```python
from build123d import *

# Parameters (mm, degrees)
BOSS_EXTRUDE1_DEPTH     = 15
SKETCH7_R               = 12.1
CUT_EXTRUDE3_DEPTH      = 71.5
SKETCH8_R               = 12.1
CUT_EXTRUDE4_DEPTH      = 71.5
CUT_EXTRUDE4_DEPTH_BACK = 71.5
BOSS_EXTRUDE4_DEPTH     = 8
BOSS_EXTRUDE5_DEPTH     = 2
SKETCH11_R              = 2.75
CUT_EXTRUDE5_DEPTH      = 24
SKETCH12_R              = 6
CUT_EXTRUDE6_DEPTH      = 4
CHAMFER1_SIZE           = 4
CUT_EXTRUDE7_DEPTH      = 28


with BuildPart() as part:
    # Sketch1 → Boss-Extrude1 (new body)
    with BuildSketch(Plane.XY):
        with BuildLine():
            Line((-23, -30.39874498), (-32, -30.39874498))
            Line((-32, -30.39874498), (-32, -39.99874498))
            Line((-32, -39.99874498), (-23, -39.99874498))
            ThreePointArc((-23, -39.99874498), (0, -46.14), (23, -39.99874498))
            Line((23, -39.99874498), (32, -39.99874498))
            Line((32, -39.99874498), (32, -30.39874498))
            Line((32, -30.39874498), (23, -30.39874498))
            Line((23, -30.39874498), (23, 39.99874498))
            ThreePointArc((23, 39.99874498), (0, 46.14), (-23, 39.99874498))
            Line((-23, 39.99874498), (-23, -30.39874498))
        make_face()
    extrude(amount=BOSS_EXTRUDE1_DEPTH)

    # Sketch7 → Cut-Extrude3 (cut)
    with BuildSketch(Plane.ZY.offset(23)):
        with Locations((0, 22.49874498)):
            Circle(SKETCH7_R)
    extrude(amount=-CUT_EXTRUDE3_DEPTH, mode=Mode.SUBTRACT)

    # Sketch8 → Cut-Extrude4 (cut, two sides)
    with BuildSketch(Plane.ZY.offset(23)) as cut_extrude4_sk:
        with Locations((0, -22.49874498)):
            Circle(SKETCH8_R)
    extrude(amount=CUT_EXTRUDE4_DEPTH, mode=Mode.SUBTRACT)
    extrude(cut_extrude4_sk.sketch, amount=-CUT_EXTRUDE4_DEPTH_BACK, mode=Mode.SUBTRACT)

    # Sketch9 → Boss-Extrude4 (add)
    with BuildSketch(Plane.ZY.offset(23)):
        with BuildLine():
            Line((0, 34.59874498), (0, 32.99874498))
            ThreePointArc((0, 32.99874498), (10.5, 22.49874498), (0, 11.99874498))
            Line((0, 11.99874498), (0, 10.39874498))
            ThreePointArc((0, 10.39874498), (12.1, 22.49874498), (0, 34.59874498))
        make_face()
    boss_extrude4 = extrude(amount=-BOSS_EXTRUDE4_DEPTH)

    # Sketch10 → Boss-Extrude5 (add)
    with BuildSketch(Plane.ZY.offset(32)):
        with BuildLine():
            Line((0, -32.99874498), (0, -34.59874498))
            ThreePointArc((0, -34.59874498), (5.040833264, -33.49874498), (9.16515139, -30.39874498))
            Line((9.16515139, -30.39874498), (6.916646586, -30.39874498))
            ThreePointArc((6.916646586, -30.39874498), (3.69459064, -32.327274881), (0, -32.99874498))
        make_face()
    boss_extrude5 = extrude(amount=-BOSS_EXTRUDE5_DEPTH)

    # Mirror1: Boss-Extrude4, Boss-Extrude5 across plane
    add(boss_extrude4.mirror(Plane(origin=(0, 0, 0), x_dir=(0, 0, 1), z_dir=(1, 0, 0))))
    add(boss_extrude5.mirror(Plane(origin=(0, 0, 0), x_dir=(0, 0, 1), z_dir=(1, 0, 0))))

    # Sketch11 → Cut-Extrude5 (cut)
    with BuildSketch(Plane(origin=(0, 0, 0), x_dir=(-1, 0, 0), z_dir=(0, 0, -1))):
        Circle(SKETCH11_R)
        with Locations((0, 41.14108798)):
            Circle(SKETCH11_R)
        with Locations((0, -41.14108798)):
            Circle(SKETCH11_R)
    extrude(amount=-CUT_EXTRUDE5_DEPTH, mode=Mode.SUBTRACT)

    # Sketch12 → Cut-Extrude6 (cut)
    with BuildSketch(Plane.XY.offset(15)):
        Circle(SKETCH12_R)
        with Locations((0, -41.14108798)):
            Circle(SKETCH12_R)
        with Locations((0, 41.14108798)):
            Circle(SKETCH12_R)
    extrude(amount=-CUT_EXTRUDE6_DEPTH, mode=Mode.SUBTRACT)

    # Chamfer1
    chamfer1_edges = [part.edges().sort_by_distance(p)[0] for p in [
        (-13.591823685, 44.092651643, 15),
        (13.591823685, 44.092651643, 15),
        (13.591823685, -44.092651643, 15),
        (27.5, -39.99874498, 15),
        (32, -39.99874498, 7.5),
        (-13.591823685, -44.092651643, 15),
        (-27.5, -39.99874498, 15),
        (-32, -39.99874498, 7.5),
    ]]
    chamfer(chamfer1_edges, length=CHAMFER1_SIZE)

    # Sketch13 → Cut-Extrude7 (cut)
    with BuildSketch(Plane.XY.offset(15)):
        Polygon((31.8, -38.311994276), (31.8, -30.59874498), (22.8, -30.59874498), (22.8, 43.889056734), (37.227618098, 33.583615236), (38.561263468, -37.220829882), align=None)
        Polygon((-37.227618098, 33.583615236), (-38.561263468, -37.220829882), (-31.8, -38.311994276), (-31.8, -30.59874498), (-22.8, -30.59874498), (-22.8, 43.889056734), align=None)
    extrude(amount=-CUT_EXTRUDE7_DEPTH, mode=Mode.SUBTRACT)


solid = part.part
```
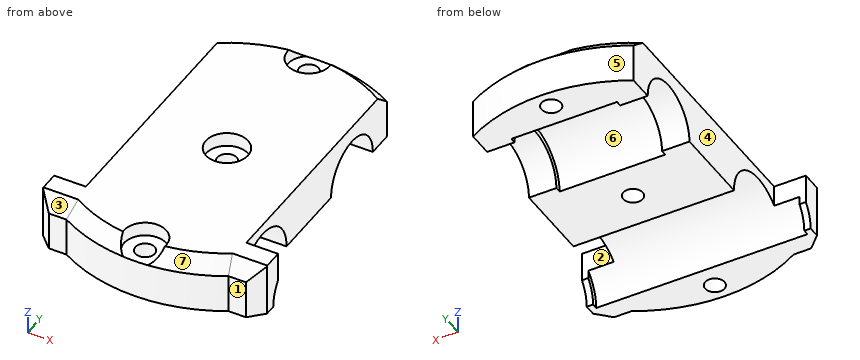
CAD build for the part. Positions are in the model's coordinates, mm. Face numbers are marked on the shaded views. A direction names the side the tool comes from. Round coordinates to 2 decimals unless told otherwise and drop trailing zeros. Loops run counter-clockwise (first coordinate to the right, second up) from the corner with the lowest first, then second, coordinate; pieces in that order, holes last. Notation, with made-up numbers: M 35,-35.5 L 59,-35.5 A21 ccw 59,-14.5 Z; hole C 4,19 d6. An arc over 180 degrees is marked long. Return JSON: item names as keys, results as strings. Group by question number.
(1) Drop flat-ended pins along their axis: P1, Ø7.5, axis at y = -2, z = 5.5, coming from the -X side; P2, Ø6.5, axis at x = 27, z = 12, coming from the +Y side; P3, Ø9, axis at x = -2.5, y = -40, coming from the +Z side; P4, Ø8, axis at y = -3, z = 12.5, coming from the +X side. Give the stop position or say it passes through.
(2) Saw through at C-C, the plane x = -24. List the corners of the cut face in (y, z), and give its area (3 significant figures).
(3) Saw through at B-B, the plane y = 0. List the corners of the cut face in (x, z).
(4) Saw through at D-D, the plane y = -28. List the corners of the cut face in (x, z).
(5) Mould opens along X. For the marked faces 5, 6 and 7 say: +X half, -X half, draft (parallel to the pull), parting line (faces both ways), or undercut.
(6) Tool access for the marked faces 1, 2, 3 and 4: list every direction of +Z, -Z, +X, -X, +Y, -Y with a clear straight run to the whole face (end or side of a thin tool).
(7) Wall check: probe 1 along X at (y, z) = (26, 10.75); probe 2 along Y at (x, z) = (0, 2.25); probe 3 along Y at (x, z) = (19, 1.25). Give the ranges that are in metal, low to high. Write a range as [from, to].
(8) Saw through at A-A, the plane x = 0. List the corners of the cut face in (y, z).
Answer list:
{
 "1": {"P1": "x = -22.8", "P2": "y = -30.6", "P3": "z = 15", "P4": "x = 22.8"},
 "2": {"outline": "M -40,0 L -34.6,0 A12.1 cw -30.6,8.99 L -30.6,15 L -36,15 L -40,11 Z", "area": "108 mm2"},
 "3": {"outline": "M -22.8,0 L -2.75,0 L -2.75,11 L -6,11 L -6,15 L -22.8,15 Z; M 2.75,0 L 22.8,0 L 22.8,15 L 6,15 L 6,11 L 2.75,11 Z"},
 "4": {"outline": "M -22.8,10.78 L 22.8,10.78 L 22.8,15 L -22.8,15 Z"},
 "5": {"face 5": "parting line", "face 6": "undercut", "face 7": "+X half"},
 "6": {"face 1": "+Z, -Z, +X, -Y", "face 2": "+Z, -Z, +X, +Y", "face 3": "+Z, -X, -Y", "face 4": "+Z, -Z, -X, +Y"},
 "7": {"probe 1": "[-22.8, -15], [15, 22.8]", "probe 2": "[-46.14, -43.89], [-38.39, -34.39], [-10.61, -2.75], [2.75, 10.61], [34.39, 38.39], [43.89, 46.14]", "probe 3": "[-42.05, -34.53], [-10.46, 12.07], [32.92, 42.05]"},
 "8": {"outline": "M -46.14,0 L -43.89,0 L -43.89,11 L -46.14,11 Z; M -38.39,0 L -34.6,0 A12.1 cw -10.4,0 L -2.75,0 L -2.75,11 L -6,11 L -6,15 L -35.14,15 L -35.14,11 L -38.39,11 Z; M 2.75,0 L 10.4,0 A12.1 cw 34.6,0 L 38.39,0 L 38.39,11 L 35.14,11 L 35.14,15 L 6,15 L 6,11 L 2.75,11 Z; M 43.89,0 L 46.14,0 L 46.14,11 L 43.89,11 Z"}
}
